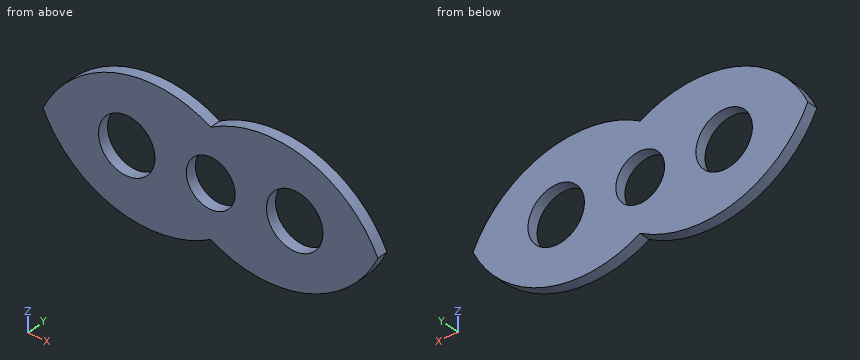
from build123d import *

# Parameters (mm, degrees)
F0_R     = 12.6
F0_R_2   = 10.9
F1_DEPTH = 5


# Not quite as in the source:
# - a feature names something its author has since deleted; it is built from what else it names


with BuildPart() as f1:
    # F0 (on Front) → F1 (new body)
    with BuildSketch(Plane.XZ):
        with BuildLine():
            ThreePointArc((74.653416872, 0), (42.4496947935, 28.0524969579), (0, 23.3572106808))
            ThreePointArc((0, 23.3572106808), (-42.5884817576, 28.1732918571), (-74.8876929283, 0))
            ThreePointArc((-74.8876929283, 0), (-42.5885090722, -28.1733794331), (0, -23.3572106808))
            ThreePointArc((0, -23.3572106808), (42.4496947935, -28.0524969579), (74.653416872, 0))
        make_face()
        with Locations((-37.5000350177, 0)):
            Circle(F0_R, mode=Mode.SUBTRACT)
        Circle(F0_R_2, mode=Mode.SUBTRACT)
        with Locations((37.5000350177, 0)):
            Circle(F0_R, mode=Mode.SUBTRACT)
    extrude(amount=F1_DEPTH)


solid = f1.part
Build history of the part. All positions in model axes, mm. Give positions to 0.01 mm unless a question says otherwise; leave off trailing zeros. Order: outer loops, then holes, each group sorted by start corner. A loop starts at its lowest first (then second) coordinate and runs counter-clockwise, first axis right, second up. Notation, with made-up numbers: M 49,-26.75 L 106,-26.75 A15 cw 106,-7.75 Z; hole C 73,22.5 d10. An arc over 180 degrees is marked long. Use one line per item in the form item = value.
1) Saw through at A-A (z = 25.5). Give the cut face in (x, y), plus the area to 3 significant figures.
Calculated:
outline = M -49.45,-5 L -4.07,-5 L -4.07,0 L -49.45,0 Z; M 4.12,-5 L 49.04,-5 L 49.04,0 L 4.12,0 Z
area = 451 mm2
2) Saw through at B-B (x = -33.5). Give the cut face in (y, z), plus the area to 3 significant figures.
Calculated:
outline = M -5,-30.16 L 0,-30.16 L 0,-11.95 L -5,-11.95 Z; M -5,11.95 L 0,11.95 L 0,30.16 L -5,30.16 Z
area = 182 mm2
3) Saw through at D-D (y = -1.15). Give the cut face in (x, z), plus the area to 3 significant figures.
Calculated:
outline = M -74.89,0 A53.16 ccw 0,-23.36 A53.16 ccw 74.65,0 A53.16 ccw 0,23.36 A53.16 ccw Z; hole C -37.5,0 d25.2; hole C 0,0 d21.8; hole C 37.5,0 d25.2
area = 5,850 mm2
4) Saw through at C-C (z = -2.5). Give the cut face in (x, y).
Calculated:
outline = M -73.63,-5 L -49.85,-5 L -49.85,0 L -73.63,0 Z; M -25.15,-5 L -10.61,-5 L -10.61,0 L -25.15,0 Z; M 10.61,-5 L 25.15,-5 L 25.15,0 L 10.61,0 Z; M 49.85,-5 L 73.39,-5 L 73.39,0 L 49.85,0 Z
5) Drop flat-ended pins along their axis: pin 1 (1 mm diameter, centred on x = 9, y = -1.5, fed in from +Z); pin 2 (1 mm diameter, centred on x = 3.5, y = -1.5, fed in from +Z); pin 3 (1.5 mm diameter, centred on x = 45.5, y = -3.5, fed in from +Z). Give the stop position or say it passes through.
Calculated:
pin_1 = 27.66
pin_2 = 25.45
pin_3 = 27.27
6) Probe probe 1 along X at (y, z) = (-3.7, -8); probe 2 along X at (y, z) = (-0.3, -8.5); probe 3 along X at (y, z) = (-2.05, 11.5). List the from-to ranges inside material, lowest first.
Calculated:
probe_1 = -70.25 to -47.23, -27.77 to -7.4, 7.4 to 27.77, 47.23 to 69.99
probe_2 = -69.89 to -46.8, -28.2 to -6.82, 6.82 to 28.2, 46.8 to 69.63
probe_3 = -67.56 to -42.65, -32.35 to 32.35, 42.65 to 67.29
